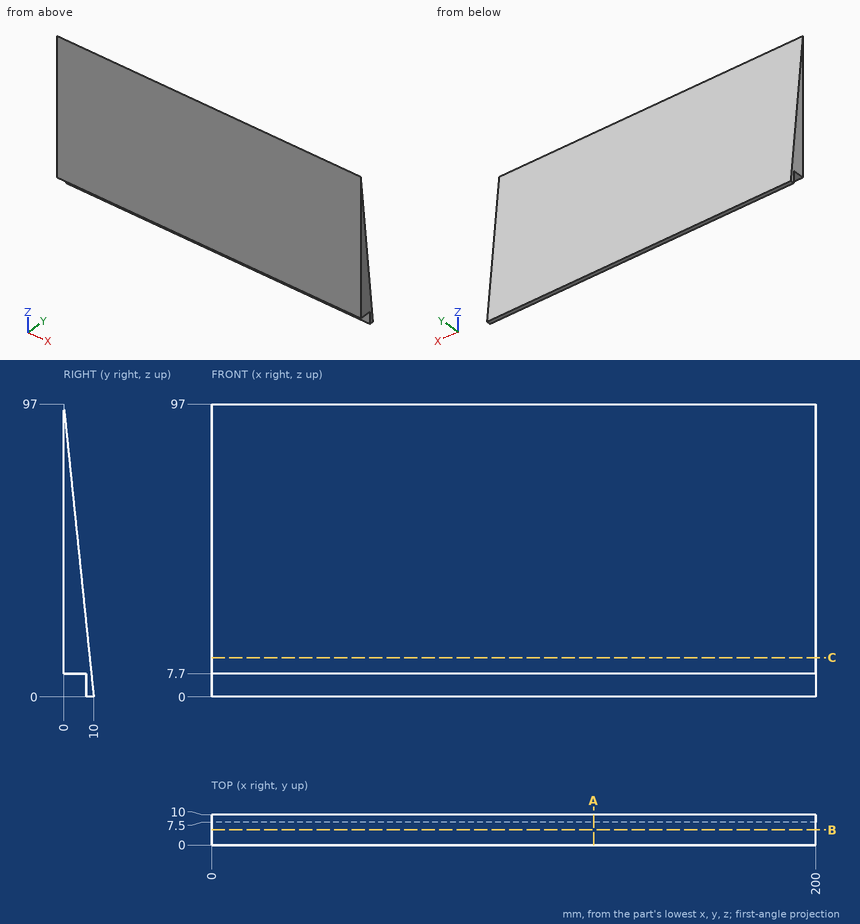
Can you work these out from the drawing? Everything is in mm from the part's minimum corner. Coordinates: 2 decimals unless noted, no trailing zeros. Loops run counter-clockwise (first coordinate to the right, second up) from the corner with the lowest first, then second, coordinate; pieces in that order, holes last.
1) Imagine slicing it at B-B (y = 5). List the corners of the cut face in (x, z) for me, and give its area (3 significant figures).
Reported:
outline: (0, 7.7) - (200, 7.7) - (200, 48.5) - (0, 48.5) - close
area: 8,160 mm2
2) Imagine slicing it at A-A (x = 126.5). List the corners of the cut face in (y, z) for me.
Reported:
outline: (0, 7.7) - (7.5, 7.7) - (7.5, 0) - (10, 0) - (0, 97) - close
3) Please list where these lines run through material, in increasing order: line 1 along Y through (x, z) = (54.5, 20.5); line 2 along Y through (x, z) = (51, 16.5).
Reported:
line 1: y = 0 to 7.89
line 2: y = 0 to 8.3
4) Will these pins go through, and if not, where does the flat tip stop? pin 1 Ø6 at (x, z) = (130, 3.5) entering from -Y; pin 2 Ø1.5 at (x, y) = (158, 6.5) entering from -Z; pin 3 Ø5 at (x, z) = (108, 61) entering from +Y.
Reported:
pin 1: stops at y = 7.5
pin 2: stops at z = 7.7
pin 3: stops at y = 3.97
5) Imagine slicing it at C-C (z = 13). List the corners of the cut face in (x, y) for me, and give its area (3 significant figures).
Reported:
outline: (0, 0) - (200, 0) - (200, 8.66) - (0, 8.66) - close
area: 1,730 mm2
